The model under review builds one solid part; all positions refer to its coordinate system, in mm. Face numbers are marked on the shaded views. A direction names the side the tool comes from. Coordinates: 2 decimals unless noted, no trailing zeros. Write each loop counter-clockwise with the first axis right and the second up, starting at its lowest first coordinate (ties: lowest second). Pieces come first, ordered by that corner, then holes. Notation, with made-up numbers: (3, 67.25) - (32, 67.25) arc R20 ccw to (32, 76.25) - close; hole circle Ø1 at (17.25, 40.5). An arc over 180 degrees is marked (long way). Put each result on its own line as item: value. Start each with the question number.
Item 1: Consider section A-A on y = 0. Give the boundary of the cut face in (x, z), then the cut area to 3 significant figures.
Item 2: Consider section B-B on x = 0. Give the boundary of the cut face in (y, z).
Item 3: For pin 1 (12 mm diameter, centred on x = 16.5, y = -38, fed in from +Z); pin 2 (1.5 mm diameter, centred on y = -6.5, z = 34, fed in from -X); pin 3 (8 mm diameter, centred on y = 21.5, z = 8, fed in from +X); pin 4 (6 mm diameter, centred on x = -32, y = -32.5, fed in from +Z), all flat-tipped, find the tip position at first contact; note any pin that passes through.
Item 4: Consider section D-D on z = -10.5. Give the boundary of the cut face in (x, y).
Item 5: To check wall thickness, follow L1, parallel to Y at x = -32, z = -53; L2, parallel to X at y = -32, z = -55; L3, parallel to Z at x = 0, y = 11. State the ranges of each line that lie inside material, in increasing order. Write a range as [from, to].
Item 6: Consider section C-C on z = 16. Give the boundary of the cut face in (x, y).
Item 7: Machinability: for the marked faces 4, 5, 6, 7 and 8, which of the approach directions +Z, -Z, +X, -X, +Y, -Y give a long, thin tool a straight path to every point of the face, cutting with its end or side? Answer none if there is none.
Item 8: Mouldability with a two-part tool opening along X and no side actions: class the marked faces 1, 2 and 3 as pulls with the +X half, pulls with the -X half, needs draft (parallel to the pull), parting line crosses it, or undercut.
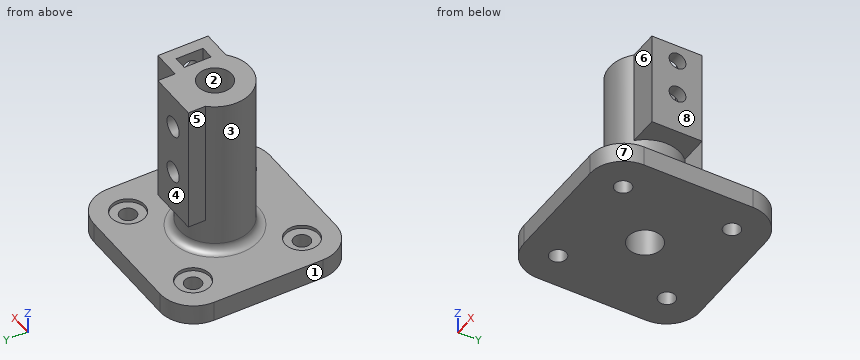
```python
from build123d import *

# Parameters (mm, degrees)
SKETCH1_R               = 21
BOSS_EXTRUDE1_DEPTH     = 48
SKETCH2_R               = 10
SKETCH2_R_2             = 5
BOSS_EXTRUDE2_DEPTH     = 12
SKETCH2_3_R             = 10
SKETCH2_3_R_2           = 5
CUT_EXTRUDE1_DEPTH      = 2
FILLET8_R               = 5
BOSS_EXTRUDE3_DEPTH     = 76
BOSS_EXTRUDE4_DEPTH     = 57
CUT_EXTRUDE2_DEPTH      = 50
SKETCH5_R               = 10
CUT_EXTRUDE3_DEPTH      = 132.059146953
CUT_EXTRUDE4_REACH      = 113.187
CUT_EXTRUDE4_END_RADIUS = 10
SKETCH6_R               = 6
CUT_EXTRUDE5_REACH      = 118.174
SKETCH7_R               = 5


with BuildPart() as part:
    # Sketch1 → Boss-Extrude1 (new, symmetric)
    with BuildSketch(Plane.XY):
        Circle(SKETCH1_R)
    extrude(amount=BOSS_EXTRUDE1_DEPTH, both=True)

    # Sketch2 → Boss-Extrude2 (add)
    # profile 1 of 10: a face of its own
    with BuildSketch(Plane(origin=(0, 0, -48), x_dir=(-1, 0, 0), z_dir=(0, 0, -1))):
        with BuildLine():
            Line((0, 52.5), (-32.5, 52.5))
            ThreePointArc((-32.5, 52.5), (-46.642135624, 46.642135624), (-52.5, 32.5))
            Line((-52.5, 32.5), (-52.5, -32.5))
            ThreePointArc((-52.5, -32.5), (-46.642135624, -46.642135624), (-32.5, -52.5))
            Line((-32.5, -52.5), (0, -52.5))
            Line((0, -52.5), (0, -21))
            ThreePointArc((0, -21), (-21, 0), (0, 21))
            Line((0, 21), (0, 52.5))
        make_face()
        with Locations((-32, -32.5)):
            Circle(SKETCH2_R, mode=Mode.SUBTRACT)
        with Locations((-32, 32.5)):
            Circle(SKETCH2_R, mode=Mode.SUBTRACT)
    # profile 2 of 10: a face of its own
    with BuildSketch(Plane(origin=(0, 0, -48), x_dir=(-1, 0, 0), z_dir=(0, 0, -1))):
        with BuildLine():
            Line((32.5, 52.5), (0, 52.5))
            Line((0, 52.5), (0, 21))
            ThreePointArc((0, 21), (14.849242405, 14.849242405), (21, 0))
            ThreePointArc((21, 0), (14.849242405, -14.849242405), (0, -21))
            Line((0, -21), (0, -52.5))
            Line((0, -52.5), (32.5, -52.5))
            ThreePointArc((32.5, -52.5), (46.642135624, -46.642135624), (52.5, -32.5))
            Line((52.5, -32.5), (52.5, 32.5))
            ThreePointArc((52.5, 32.5), (46.642135624, 46.642135624), (32.5, 52.5))
        make_face()
        with Locations((32, -32.5)):
            Circle(SKETCH2_R, mode=Mode.SUBTRACT)
        with Locations((32, 32.5)):
            Circle(SKETCH2_R, mode=Mode.SUBTRACT)
    # profile 3 of 10: a face of its own
    with BuildSketch(Plane(origin=(0, 0, -48), x_dir=(-1, 0, 0), z_dir=(0, 0, -1))):
        with Locations((-32, 32.5)):
            Circle(SKETCH2_R)
        with Locations((-32, 32.5)):
            Circle(SKETCH2_R_2, mode=Mode.SUBTRACT)
    # profile 4 of 10: a face of its own
    with BuildSketch(Plane(origin=(0, 0, -48), x_dir=(-1, 0, 0), z_dir=(0, 0, -1))):
        with Locations((-32, -32.5)):
            Circle(SKETCH2_R)
        with Locations((-32, -32.5)):
            Circle(SKETCH2_R_2, mode=Mode.SUBTRACT)
    # profile 5 of 10: a face of its own
    with BuildSketch(Plane(origin=(0, 0, -48), x_dir=(-1, 0, 0), z_dir=(0, 0, -1))):
        with Locations((32, 32.5)):
            Circle(SKETCH2_R)
        with Locations((32, 32.5)):
            Circle(SKETCH2_R_2, mode=Mode.SUBTRACT)
    # profile 6 of 10: a face of its own
    with BuildSketch(Plane(origin=(0, 0, -48), x_dir=(-1, 0, 0), z_dir=(0, 0, -1))):
        with Locations((32, -32.5)):
            Circle(SKETCH2_R)
        with Locations((32, -32.5)):
            Circle(SKETCH2_R_2, mode=Mode.SUBTRACT)
    # profile 7 of 10: a face of its own
    with BuildSketch(Plane(origin=(0, 0, -48), x_dir=(-1, 0, 0), z_dir=(0, 0, -1))):
        with BuildLine():
            ThreePointArc((21, 0), (14.849242405, 14.849242405), (0, 21))
            Line((0, 21), (0, -21))
            ThreePointArc((0, -21), (14.849242405, -14.849242405), (21, 0))
        make_face()
    # profile 8 of 10: a face of its own
    with BuildSketch(Plane(origin=(0, 0, -48), x_dir=(-1, 0, 0), z_dir=(0, 0, -1))):
        with BuildLine():
            Line((0, -21), (0, 21))
            ThreePointArc((0, 21), (-21, 0), (0, -21))
        make_face()
    # profile 9 of 10: a face of its own
    with BuildSketch(Plane(origin=(0, 0, -48), x_dir=(-1, 0, 0), z_dir=(0, 0, -1))):
        with BuildLine():
            ThreePointArc((21, 0), (14.849242405, 14.849242405), (0, 21))
            Line((0, 21), (0, -21))
            ThreePointArc((0, -21), (14.849242405, -14.849242405), (21, 0))
        make_face()
    # profile 10 of 10: a face of its own
    with BuildSketch(Plane(origin=(0, 0, -48), x_dir=(-1, 0, 0), z_dir=(0, 0, -1))):
        with BuildLine():
            Line((0, -21), (0, 21))
            ThreePointArc((0, 21), (-21, 0), (0, -21))
        make_face()
    extrude(amount=BOSS_EXTRUDE2_DEPTH)

    # Sketch2<3> → Cut-Extrude1 (cut)
    # profile 1 of 4: a face of its own
    with BuildSketch(Plane(origin=(0, 0, -48), x_dir=(-1, 0, 0), z_dir=(0, 0, -1))):
        with Locations((32, 32.5)):
            Circle(SKETCH2_3_R)
        with Locations((32, 32.5)):
            Circle(SKETCH2_3_R_2, mode=Mode.SUBTRACT)
    # profile 2 of 4: a face of its own
    with BuildSketch(Plane(origin=(0, 0, -48), x_dir=(-1, 0, 0), z_dir=(0, 0, -1))):
        with Locations((-32, 32.5)):
            Circle(SKETCH2_3_R)
        with Locations((-32, 32.5)):
            Circle(SKETCH2_3_R_2, mode=Mode.SUBTRACT)
    # profile 3 of 4: a face of its own
    with BuildSketch(Plane(origin=(0, 0, -48), x_dir=(-1, 0, 0), z_dir=(0, 0, -1))):
        with Locations((-32, -32.5)):
            Circle(SKETCH2_3_R)
        with Locations((-32, -32.5)):
            Circle(SKETCH2_3_R_2, mode=Mode.SUBTRACT)
    # profile 4 of 4: a face of its own
    with BuildSketch(Plane(origin=(0, 0, -48), x_dir=(-1, 0, 0), z_dir=(0, 0, -1))):
        with Locations((32, -32.5)):
            Circle(SKETCH2_3_R)
        with Locations((32, -32.5)):
            Circle(SKETCH2_3_R_2, mode=Mode.SUBTRACT)
    extrude(amount=CUT_EXTRUDE1_DEPTH, mode=Mode.SUBTRACT)

    # Fillet8
    fillet8_edges = [part.edges().sort_by_distance(p)[0] for p in [
        (-21, 0, -48),
    ]]
    fillet(fillet8_edges, radius=FILLET8_R)

    # Sketch3 → Boss-Extrude3 (add)
    with BuildSketch(Plane.XY.offset(48)):
        with BuildLine():
            Line((-15, 25), (15, 25))
            Line((15, 25), (15, 14.696938457))
            ThreePointArc((15, 14.696938457), (0, 21), (-15, 14.696938457))
            Line((-15, 14.696938457), (-15, 25))
        make_face()
    extrude(amount=-BOSS_EXTRUDE3_DEPTH)

    # Sketch4 → Boss-Extrude4 (add)
    with BuildSketch(Plane.XY.offset(48)):
        with BuildLine():
            Line((32, 14.696938457), (15, 14.696938457))
            ThreePointArc((15, 14.696938457), (20.995532794, -0.433131267), (14.381109394, -15.303061543))
            Line((14.381109394, -15.303061543), (32, -15.303061543))
            Line((32, -15.303061543), (32, 14.696938457))
        make_face()
    extrude(amount=-BOSS_EXTRUDE4_DEPTH)

    # Sketch4<3> → Cut-Extrude2 (cut)
    with BuildSketch(Plane.XY.offset(48)):
        with BuildLine():
            ThreePointArc((19.416487839, -8), (21, 0), (19.416487839, 8))
            Line((19.416487839, 8), (17, 8))
            Line((17, 8), (17, -8))
            Line((17, -8), (19.416487839, -8))
        make_face()
        with BuildLine():
            Line((25, 8), (19.416487839, 8))
            ThreePointArc((19.416487839, 8), (21, 0), (19.416487839, -8))
            Line((19.416487839, -8), (25, -8))
            Line((25, -8), (25, 8))
        make_face()
    extrude(amount=-CUT_EXTRUDE2_DEPTH, mode=Mode.SUBTRACT)

    # Sketch5 → Cut-Extrude3 (cut, through all)
    with BuildSketch(Plane.XY.offset(48)):
        Circle(SKETCH5_R)
    extrude(amount=-CUT_EXTRUDE3_DEPTH, mode=Mode.SUBTRACT)

    # Cut-Extrude4: up to this cylinder (the profile starts outside it)
    cut_extrude4_end = Plane(origin=(0, 0, 13), z_dir=(0, 0, 1)) * Cylinder(CUT_EXTRUDE4_END_RADIUS, 277.374, mode=Mode.PRIVATE)
    # Sketch6 → Cut-Extrude4 (cut, up to the surface)
    with BuildSketch(Plane(origin=(0, 25, 0), x_dir=(1, 0, 0), z_dir=(0, 1, 0)), mode=Mode.PRIVATE) as cut_extrude4_sk1:
        with Locations(Location((0, 2, 0), (0, 0, 270))):
            Circle(SKETCH6_R)
    cut_extrude4_tool1 = extrude(cut_extrude4_sk1.sketch, amount=-CUT_EXTRUDE4_REACH, mode=Mode.PRIVATE) - cut_extrude4_end
    add(cut_extrude4_tool1.solids().sort_by_distance((0, 25, -2))[0], mode=Mode.SUBTRACT)
    # Sketch6 → Cut-Extrude4 (cut, up to the surface)
    with BuildSketch(Plane(origin=(0, 25, 0), x_dir=(1, 0, 0), z_dir=(0, 1, 0)), mode=Mode.PRIVATE) as cut_extrude4_sk2:
        with Locations(Location((0, -28, 0), (0, 0, 270))):
            Circle(SKETCH6_R)
    cut_extrude4_tool2 = extrude(cut_extrude4_sk2.sketch, amount=-CUT_EXTRUDE4_REACH, mode=Mode.PRIVATE) - cut_extrude4_end
    add(cut_extrude4_tool2.solids().sort_by_distance((0, 25, 28))[0], mode=Mode.SUBTRACT)

    # Sketch7 → Cut-Extrude5 (cut, up to next)
    with BuildSketch(Plane(origin=(32, 0, 0), x_dir=(0, 0, -1), z_dir=(1, 0, 0)), mode=Mode.PRIVATE) as cut_extrude5_sk1:
        with Locations(Location((-38, 0, 0), (0, 0, 90))):
            Circle(SKETCH7_R)
    cut_extrude5_tool1 = extrude(cut_extrude5_sk1.sketch, amount=-CUT_EXTRUDE5_REACH, mode=Mode.PRIVATE) & part.part
    # Sketch7 → Cut-Extrude5 (cut, up to next)
    with BuildSketch(Plane(origin=(32, 0, 0), x_dir=(0, 0, -1), z_dir=(1, 0, 0)), mode=Mode.PRIVATE) as cut_extrude5_sk2:
        with Locations(Location((-16, 0, 0), (0, 0, 90))):
            Circle(SKETCH7_R)
    cut_extrude5_tool2 = extrude(cut_extrude5_sk2.sketch, amount=-CUT_EXTRUDE5_REACH, mode=Mode.PRIVATE) & part.part
    add(cut_extrude5_tool1.solids().sort_by_distance((32, 0, 38))[0], mode=Mode.SUBTRACT)
    add(cut_extrude5_tool2.solids().sort_by_distance((32, 0, 16))[0], mode=Mode.SUBTRACT)


solid = part.part
```
Report:
1. outline: (-52.5, -60) - (-10, -60) - (-10, 48) - (-21, 48) - (-21, -43) arc R5 cw to (-26, -48) - (-52.5, -48) - close; (10, -60) - (52.5, -60) - (52.5, -48) - (26, -48) arc R5 cw to (21, -43) - (21, -9) - (32, -9) - (32, 11) - (25, 11) - (25, -2) - (17, -2) - (17, 48) - (10, 48) - close; (25, 21) - (32, 21) - (32, 33) - (25, 33) - close; (25, 43) - (32, 43) - (32, 48) - (25, 48) - close
1. area: 3,230 mm²
2. outline: (-52.5, -60) - (-10, -60) - (-10, 48) - (-21, 48) - (-21, -43) arc R5 cw to (-26, -48) - (-52.5, -48) - close; (10, -60) - (52.5, -60) - (52.5, -48) - (26, -48) arc R5 cw to (21, -43) - (21, -28) - (25, -28) - (25, -8) - (10, -8) - close; (10, 4) - (25, 4) - (25, 22) - (10, 22) - close; (10, 34) - (25, 34) - (25, 48) - (10, 48) - close
3. pin 1: z = -48
3. pin 2: x = -20.2
3. pin 3: x = 15
3. pin 4: through
4. outline: (-15, 14.7) arc R21 ccw (long way) to (15, 14.7) - (15, 25) - (-15, 25) - close; hole circle Ø20 at (0, 0)
5. L1: [-52.5, -37.5], [-27.5, 27.5], [37.5, 52.5]
5. L2: [-52.5, -36.97], [-27.03, 27.03], [36.97, 52.5]
5. L3: [-60, -8], [4, 22], [34, 48]
6. outline: (-15, 14.7) arc R21 ccw to (14.38, -15.3) - (32, -15.3) - (32, -5) - (25, -5) - (25, -8) - (17, -8) - (17, 8) - (25, 8) - (25, 5) - (32, 5) - (32, 14.7) - (15, 14.7) - (15, 25) - (-15, 25) - close; hole circle Ø20 at (0, 0)
7. face 4: +Z, +X, -X, +Y
7. face 5: +Z, -X, +Y
7. face 6: +Z, +X, -Y
7. face 7: +Z, -Z, +X, -Y
7. face 8: +Z, +X, +Y, -Y
8. face 1: pulls with the -X half
8. face 2: undercut
8. face 3: parting line crosses it
